from build123d import *

# Parameters (mm, degrees)
PAD001_DEPTH    = 60
SKETCH003_R     = 65
POCKET001_DEPTH = 20
POCKET003_DEPTH = 39
SKETCH015_R     = 3
POCKET004_DEPTH = 40.001


with BuildPart() as part:
    # Sketch002 → Pad001 (new body)
    with BuildSketch(Plane.XY):
        Polygon((49, 84.87049), (-49, 84.87049), (-98, 0), (-49, -84.87049), (49, -84.87049), (98, 0), align=None)
    extrude(amount=PAD001_DEPTH)

    # Sketch003 (on Face8 of Pad001) → Pocket001 (cut)
    with BuildSketch(Plane.XY.offset(60)):
        Circle(SKETCH003_R)
    extrude(amount=-POCKET001_DEPTH, mode=Mode.SUBTRACT)

    # Sketch014 (on Face4 of Pocket001) → Pocket003 (cut)
    with BuildSketch(Plane(origin=(0, 0, 0), x_dir=(1, 0, 0), z_dir=(0, 0, -1))):
        Polygon((44.381198, 76.87049), (-44.381198, 76.87049), (-88.762396, 0), (-44.381198, -76.87049), (44.381198, -76.87049), (88.762396, 0), align=None)
    extrude(amount=-POCKET003_DEPTH, mode=Mode.SUBTRACT)

    # Sketch015 (on Face17 of Pocket003) → Pocket004 (cut, through all)
    with BuildSketch(Plane.XY.offset(40)):
        Circle(SKETCH015_R)
    extrude(amount=-POCKET004_DEPTH, mode=Mode.SUBTRACT)


solid = part.part
Design review of the part built by this model. Coordinates are the model's own, in mm. A direction names the side the tool comes from. Round coordinates to 2 decimals unless told otherwise and drop trailing zeros. Write each loop counter-clockwise with the first axis right and the second up, starting at its lowest first coordinate (ties: lowest second). Pieces come first, ordered by that corner, then holes.
Item 1: Consider section D-D on y = -61. Give the boundary of the cut face in (x, z), and give its area (3 significant figures).
Item 2: Consider section B-B on z = 46. Give the boundary of the cut face in (x, y).
Item 3: Draft analysis for pull direction Y (two halves, no side actions). For faces 4 (the flat face through (73.843, 41.841, 29.58)), 5 (the flat face through (66.261, 38.973, 19.227)), 6 (the flat face through (-73.843, -41.841, 29.58)), state which applies: released by +Y, released by -Y, zero draft, split by the parting line, or undercut.
Item 4: Consider section A-A on x = 0. Give the boundary of the cut face in (y, z), and give its area (3 significant figures).
Item 5: For faces 1 (the flat face through (-1, 76.87, 19)), 2 (the flat face through (1, 84.87, 30)), 3 (the flat face through (14, 1, 40)), list the 3-axis set-ups (+Z, -Z, +X, -X, +Y, -Y) from which the entire face can be reached by the end or side of a thin tool; tool diameter is ignored.
Item 6: Wall thickness on L1, parallel to Y at x = 0, z = 49; L2, parallel to Z at x = -60, y = 2; L3, parallel to Z at x = 31, y = -65.5: over which ranges is each line inside the solid? List them lowest first.
Item 7: For pin 1 Ø1 at (x, z) = (-52, 32.5) entering from -Y; pin 2 Ø2 at (y, z) = (-41.5, 19) entering from +X; pin 3 Ø6 at (y, z) = (-53, 52) entering from +X, all flat-tipped, find the tip position at first contact; note any pin that passes through.
Item 8: Consider section C-C on x = 68. Give the boundary of the cut face in (y, z).
Check values:
1. outline: (-62.78, 0) - (-53.54, 0) - (-53.54, 39) - (53.54, 39) - (53.54, 0) - (62.78, 0) - (62.78, 60) - (22.45, 60) - (22.45, 40) - (-22.45, 40) - (-22.45, 60) - (-62.78, 60) - close
1. area: 2,460 mm2
2. outline: (-98, 0) - (-49, -84.87) - (49, -84.87) - (98, 0) - (49, 84.87) - (-49, 84.87) - close; hole circle Ø130 at (0, 0)
3. face 4: released by +Y
3. face 5: undercut
3. face 6: released by -Y
4. outline: (-84.87, 0) - (-76.87, 0) - (-76.87, 39) - (-3, 39) - (-3, 40) - (-65, 40) - (-65, 60) - (-84.87, 60) - close; (3, 39) - (76.87, 39) - (76.87, 0) - (84.87, 0) - (84.87, 60) - (65, 60) - (65, 40) - (3, 40) - close
4. area: 1,580 mm2
5. face 1: -Z
5. face 2: +Z, -Z, +X, -X, +Y
5. face 3: +Z
6. L1: y = -84.87 to -65, 65 to 84.87
6. L2: z = 39 to 40
6. L3: z = 39 to 60
7. pin 1: stops at y = -80.54
7. pin 2: stops at x = 74.62
7. pin 3: stops at x = 69.13
8. outline: (-51.96, 0) - (-35.96, 0) - (-35.96, 39) - (35.96, 39) - (35.96, 0) - (51.96, 0) - (51.96, 60) - (-51.96, 60) - close
